Autodesk Inventor part; units mm, degrees
ref_plane "YZ Plane" through (0, 0, 0) normal (1, 0, 0) x (0, 1, 0)
ref_plane "XZ Plane" through (0, 0, 0) normal (0, 1, 0) x (-1, 0, 0)
ref_plane "XY Plane" through (0, 0, 0) normal (0, 0, 1) x (1, 0, 0)
sketch "Sketch1" plane through (0, 0, 0) normal (1, 0, 0) x (0, 1, 0)
  circle A0 centre (0, 0) radius 62.5 construction
  circle A1 centre (-146.0656, -2.5) radius 50 construction
  line L0 (-146.0656, -2.5) -> (0, 0) construction
  line L1 (-172.7208, -52.5) -> (-113.4241, -52.5) construction
  line L2 (-16.0459, -62.5) -> (40.9165, -62.5) construction
  line L3 (-162.86, -17.263) -> (-144.3319, -24.7934)
  line L4 (-144.3319, -24.7934) -> (-74.6779, -21.7515)
  line L5 (42.063, -16.6532) -> (72.2375, 41.3128)
  line L6 (72.2375, 41.3128) -> (-2.0558, 79.9865)
  line L7 (-2.0558, 79.9865) -> (-145.8225, 73.708)
  line L8 (-145.8225, 73.708) -> (-182.9035, 44.86)
  line L9 (-182.9035, 44.86) -> (-162.86, -17.263)
  circle A2 centre (0, 0) radius 16.3
  circle A3 centre (-146.0656, -2.5) radius 12.2
  line L10 (-153.5959, -21.0282) -> (-146.0656, -2.5) construction
  arc A4 (-63.375, -21.2579) -> (-74.6779, -21.7515) centre (-69.3319, -14.5113) ccw construction
  line L11 (-99.9551, -22.8554) -> (-99.3168, -22.8275) construction
  line L12 (-99.3168, -22.8275) -> (-63.375, -21.2579) construction
  line L13 (-63.375, -21.2579) -> (-99.9551, -22.8554) construction
  line L14 (-74.6779, -21.7515) -> (42.063, -16.6532)
  line L15 (0, 0) -> (-212.6616, 0) construction
  circle A5 centre (-86.0656, 0.7731) radius 4.25
  dimension "d0" = 125
  dimension "d1" = 100
  dimension "d2" = 146.087
  dimension "d3" = 10
  dimension "d4" = 20
  dimension "d5" = 32.6
  dimension "d6" = 24.4
  dimension "d7" = 23.099
  dimension "d8" = 20
  dimension "d9" = 130
  dimension "d10" = 110
  dimension "d12" = 155.381
  dimension "d13" = 80
  dimension "d14" = 90
  dimension "d15" = 150
  dimension "Height" = 70
  dimension "d17" = 45
  dimension "d18" = 60
  dimension "d30" = 8.5
  dimension "d31" = 23
  dimension "d32" = 60
extrude "Extrusion1" add sketch "Sketch1" along normal blind 4
fillet "Fillet3" radius 10 6 edges at (2, 72.2375, 41.3128) (2, 42.063, -16.6532) (2, -144.3319, -24.7934) (2, -162.86, -17.263) (2, -182.9035, 44.86) (2, -145.8225, 73.708)
chamfer "Chamfer1" distance 32 angle 45 1 edges at (2, -2.0558, 79.9865)
fillet "Fillet4" radius 10 2 edges at (2, 26.3287, 65.2108) (2, -34.0253, 78.5903)
sketch "Sketch2" plane through (4, 0, 0) normal (1, 0, 0) x (0, 0, -1)
  circle A0 centre (0, 0) radius 16.3
  circle A1 centre (0, 0) radius 16.3
  circle A2 centre (-62.3406, -136.0055) radius 4.25
  line L0 (-71.7494, -148.34) -> (-49.1595, -177.377)
  line L1 (-38.1961, -180.7535) -> (12.8252, -164.2919)
  circle A3 centre (-37.9106, 61.4474) radius 4.25
  arc A4 (-32.4427, 67.6201) -> (-45.9302, 63.3673) centre (-37.0601, 58.7499) ccw
  line L2 (11.532, 44.7289) -> (-32.4427, 67.6201)
  line L3 (-45.9302, 63.3673) -> (-64.6029, 27.4965)
  circle A5 centre (-55.1197, -61.0055) radius 4.25
  line L4 (-55.1197, -61.0055) -> (-62.3406, -136.0055)
  line L5 (-78.5329, -35.3406) -> (-73.8471, -142.6359)
  point P0 (18.0192, 10.7846)
  point P1 (18.8908, -9.1727)
  dimension "d39" = 32.6
  dimension "d42" = 8.5
  dimension "d43" = 15
  dimension "d44" = 50
  dimension "d45" = 8.5
  dimension "d47" = 8
  dimension "d48" = 8
  dimension "d49" = 8.5
  dimension "d50" = 8
  dimension "d51" = 75
extrude "Extrusion2" cut sketch "Sketch2" against normal blind 9.5
properties part number "Module Plate 1" material "Aluminum 6061"
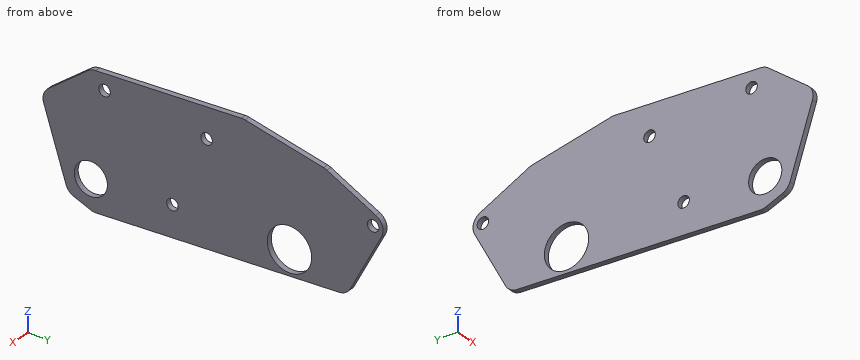
Check sheet for the modelled part. Datum: model origin and axes. Units: mm. Give positions to 0.01 mm unless a question says otherwise; leave off trailing zeros. Loops run counter-clockwise (first coordinate to the right, second up) from the corner with the lowest first, then second, coordinate; pieces in that order, holes last. Notation, with made-up numbers: M -14,-4.5 L 21,-4.5 A22 cw 21,26.5 Z; hole C 54,64.25 d1. An arc over 180 degrees is marked long. Return JSON: item names as keys, results as strings. Group by question number.
1. Cross-section at D-D on z = -8. Record the boundary of the cut face in (x, y).
2. Go/stop test with a flat-tipped pin: pin 1 (2 mm diameter, centred on x = 3.5, z = -10.5, fed in from +Y). Record where the tip stops, or that it passes through.
3. Cross-section at A-A on y = -154. Record the boundary of the cut face in (x, z), plus the area to 3 significant figures.
4. Cross-section at C-C on x = 2. State how many separate pieces and enclosed holes the cut face has, plus the area to 3 significant figures.
5. Cross-section at B-B on z = 12. Record the boundary of the cut face in (x, y), plus the area to 3 significant figures.
6. Thickness scan on L1, parallel to Y at x = 3.5, z = -12; L2, parallel to Y at x = 0.85, z = 12; L3, parallel to Y at x = 2.7, z = -9. Record the ranges inside material, lowest first.
Return value:
{
 "1": {"outline": "M 0,-165.85 L 4,-165.85 L 4,-156.96 L 0,-156.96 Z; M 0,-135.18 L 4,-135.18 L 4,-14.2 L 0,-14.2 Z; M 0,14.2 L 4,14.2 L 4,46.57 L 0,46.57 Z"},
 "2": {"pin 1": "y = 45.79"},
 "3": {"outline": "M 0,-20.86 L 4,-20.86 L 4,-11.77 L 0,-11.77 Z; M 0,6.77 L 4,6.77 L 4,67.35 L 0,67.35 Z", "area": "279 mm^2"},
 "4": {"separate pieces": "1", "enclosed holes": "6", "area": "19,500 mm^2"},
 "5": {"outline": "M 0,-172.3 L 4,-172.3 L 4,-11.03 L 0,-11.03 Z; M 0,11.03 L 4,11.03 L 4,56.98 L 0,56.98 Z", "area": "829 mm^2"},
 "6": {"L1": "-164.56 to -153.72, -138.41 to -11.03, 11.03 to 44.47", "L2": "-172.3 to -11.03, 11.03 to 56.98", "L3": "-165.53 to -156.39, -135.74 to -13.59, 13.59 to 46.05"}
}
